Work out the finished part from the listing and answer in its coordinate system (mm). Give positions to 0.01 mm unless a question says otherwise; leave off trailing zeros. Write each loop counter-clockwise with the first axis right and the second up, starting at its lowest first coordinate (ties: lowest second). Pieces come first, ordered by that corner, then holes. Notation, with made-up numbers: (86.5, -16) -> (133.5, -16) arc R20 ccw to (133.5, 22) -> close; hole circle Ø10 at (-3, 8.5). An arc over 180 degrees is marked (long way). Use a Markdown table: item, result. Add a question column.
Q1. Section C-C, the plane y = 2.2 is taken. State how many separate pieces and enclosed holes the cut face has, plus the area to 3 significant figures.
Q2. Section B-B, the plane x = 25 is taken. Give the vertices of the cut face in (y, z).
Q3. Section A-A, the plane z = 2.5 is taken. Give the vertices of the cut face in (x, y) (3 decimals), plus the area to 3 significant figures.
Q4. Consider line 1 (X direction, y = 1.7, z = -28.5); line 2 (X direction, y = 2.55, z = -1.5) (3 decimals); line 3 (Z direction, x = 25.5, y = 3.35). Determine where each line is inside the solid, lowest interval first.
Q5. This flat-tipped pin is pushed along its axis until it touches: pin 1 Ø1.1 at (x, y) = (111.5, 2.5) entering from +Z. Where does it stop, or does it pass through?
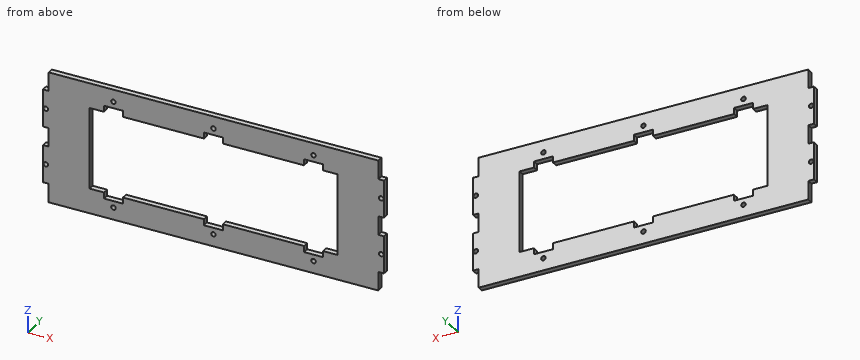
from build123d import *

# Parameters (mm, degrees)
SKETCH1_R           = 1.524
BOSS_EXTRUDE1_DEPTH = 3.81


with BuildPart() as part:
    # Sketch1 → Boss-Extrude1 (new body)
    with BuildSketch(Plane(origin=(0, 0, 0), x_dir=(1, 0, 0), z_dir=(0, 1, 0))):
        Polygon((-110.49, -44.45), (110.49, -44.45), (110.49, -31.75), (114.3, -31.75), (114.3, -6.35), (110.49, -6.35), (110.49, 6.35), (114.3, 6.35), (114.3, 31.75), (110.49, 31.75), (110.49, 44.45), (-110.49, 44.45), (-110.49, 31.75), (-114.3, 31.75), (-114.3, 6.35), (-110.49, 6.35), (-110.49, -6.35), (-114.3, -6.35), (-114.3, -31.75), (-110.49, -31.75), align=None)
        with Locations((112.395, 19.05)):
            Circle(SKETCH1_R, mode=Mode.SUBTRACT)
        with Locations((-112.395, 19.05)):
            Circle(SKETCH1_R, mode=Mode.SUBTRACT)
        with Locations((-112.395, -19.05)):
            Circle(SKETCH1_R, mode=Mode.SUBTRACT)
        with Locations((112.395, -19.05)):
            Circle(SKETCH1_R, mode=Mode.SUBTRACT)
        with Locations((-67.056, -36.195)):
            Circle(SKETCH1_R, mode=Mode.SUBTRACT)
        with Locations((0, -36.195)):
            Circle(SKETCH1_R, mode=Mode.SUBTRACT)
        with Locations((67.056, -36.195)):
            Circle(SKETCH1_R, mode=Mode.SUBTRACT)
        with Locations((67.056, 36.195)):
            Circle(SKETCH1_R, mode=Mode.SUBTRACT)
        with Locations((-67.056, 36.195)):
            Circle(SKETCH1_R, mode=Mode.SUBTRACT)
        with Locations((0, 36.195)):
            Circle(SKETCH1_R, mode=Mode.SUBTRACT)
        Polygon((-83.185, -27.5844), (-73.406, -27.5844), (-73.406, -31.75), (-60.706, -31.75), (-60.706, -27.5844), (-6.35, -27.5844), (-6.35, -31.75), (6.35, -31.75), (6.35, -27.5844), (60.706, -27.5844), (60.706, -31.75), (73.406, -31.75), (73.406, -27.5844), (83.185, -27.5844), (83.185, 27.5844), (73.406, 27.5844), (73.406, 31.75), (60.706, 31.75), (60.706, 27.5844), (6.35, 27.5844), (6.35, 31.75), (-6.35, 31.75), (-6.35, 27.5844), (-60.706, 27.5844), (-60.706, 31.75), (-73.406, 31.75), (-73.406, 27.5844), (-83.185, 27.5844), align=None, mode=Mode.SUBTRACT)
    extrude(amount=BOSS_EXTRUDE1_DEPTH)


solid = part.part
Result set:
| question | item | result |
|---|---|---|
| 1 | separate pieces | 1 |
| 1 | enclosed holes | 11 |
| 1 | area | 10,500 mm2 |
| 2 | outline | (0, -44.45) -> (3.81, -44.45) -> (3.81, -27.58) -> (0, -27.58) -> close; (0, 27.58) -> (3.81, 27.58) -> (3.81, 44.45) -> (0, 44.45) -> close |
| 3 | outline | (-110.49, 0) -> (-83.185, 0) -> (-83.185, 3.81) -> (-110.49, 3.81) -> close; (83.185, 0) -> (110.49, 0) -> (110.49, 3.81) -> (83.185, 3.81) -> close |
| 3 | area | 208 mm2 |
| 4 | line 1 | x = -114.3 to -73.41, -60.71 to -6.35, 6.35 to 60.71, 73.41 to 114.3 |
| 4 | line 2 | x = -110.49 to -83.185, 83.185 to 110.49 |
| 4 | line 3 | z = -44.45 to -27.58, 27.58 to 44.45 |
| 5 | pin 1 | stops at z = 31.75 |
